```python
from build123d import *

# Parameters (mm, degrees)
SKETCH_1_W           = 58.5
SKETCH_1_H           = 40
EXTRUDE_1_DEPTH      = 25
SKETCH_2_OUTSIDE_W   = 75.53
SKETCH_2_OUTSIDE_H   = 57.03
SKETCH_2_OUTSIDE_W_2 = 51.5
SKETCH_2_OUTSIDE_H_2 = 31.5
CUT_EXTRUDE_4_DEPTH  = 21.5
EXTRUDE_2_REACH      = 45.365
SKETCH_3_W           = 3.457860742
SKETCH_3_H           = 3.97738732
FILLET_1_R           = 3
FILLET_2_R           = 3
FILLET_3_R           = 3


with BuildPart() as part:
    # 草图1 → 凸台-拉伸1 (new body)
    with BuildSketch(Plane.XY):
        Rectangle(SKETCH_1_W, SKETCH_1_H)
    extrude(amount=EXTRUDE_1_DEPTH)

    # 草图2 outside → 切除-拉伸4 (cut)
    with BuildSketch(Plane.XY.offset(25)):
        Rectangle(SKETCH_2_OUTSIDE_W, SKETCH_2_OUTSIDE_H)
        Rectangle(SKETCH_2_OUTSIDE_W_2, SKETCH_2_OUTSIDE_H_2, mode=Mode.SUBTRACT)
    extrude(amount=-CUT_EXTRUDE_4_DEPTH, mode=Mode.SUBTRACT)

    # 草图3 → 凸台-拉伸2 (add, up to next)
    with BuildSketch(Plane.XY.offset(25), mode=Mode.PRIVATE) as extrude_2_sk1:
        with Locations((25.75, 0)):
            Rectangle(SKETCH_3_W, SKETCH_3_H)
    extrude_2_tool1 = extrude(extrude_2_sk1.sketch, amount=-EXTRUDE_2_REACH, mode=Mode.PRIVATE) - part.part
    add(extrude_2_tool1.solids().sort_by_distance((25.75, 0, 25))[0])

    # 圆角1
    fillet_1_edges = [part.edges().sort_by_distance(p)[0] for p in [
        (25.75, -15.75, 14.25),
        (25.75, 15.75, 14.25),
    ]]
    fillet(fillet_1_edges, radius=FILLET_1_R)

    # 圆角2
    fillet_2_edges = [part.edges().sort_by_distance(p)[0] for p in [
        (-25.75, -15.75, 14.25),
        (-25.75, 15.75, 14.25),
    ]]
    fillet(fillet_2_edges, radius=FILLET_2_R)

    # 圆角3
    fillet_3_edges = [part.edges().sort_by_distance(p)[0] for p in [
        (29.25, -20, 1.75),
        (-29.25, -20, 1.75),
        (-29.25, 20, 1.75),
        (29.25, 20, 1.75),
    ]]
    fillet(fillet_3_edges, radius=FILLET_3_R)


solid = part.part
```
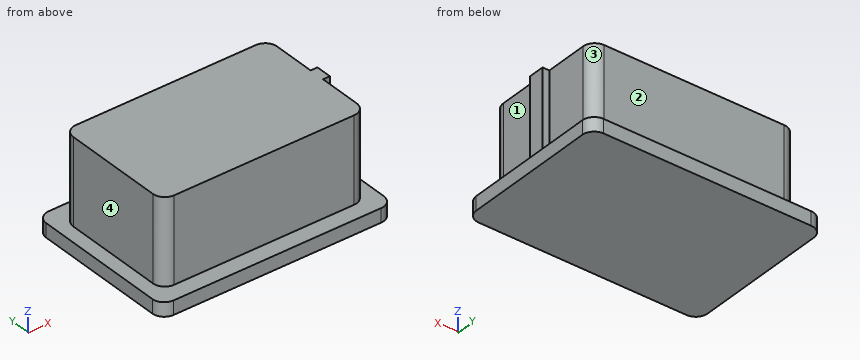
Geometry check sheet. Reference: the model listing, model coordinates, mm. Face numbers are marked on the shaded views. A direction names the side the tool comes from. Coordinates: 2 decimals unless noted, no trailing zeros. Order: outer loops, then holes, each group sorted by start corner. A loop starts at its lowest first (then second) coordinate and runs counter-clockwise, first axis right, second up. Notation, with made-up numbers: (7, 65.5) - (30, 65.5) arc R8 cw to (30, 72.5) - close; hole circle Ø4 at (83, 89). An arc over 180 degrees is marked (long way). Answer in a Markdown table with one row per item. Add a question column.
1. Section check C-C (z = 4.25). Enter the section's corners in (x, y).
2. Material ranges on L1, parallel to Z at x = -26, y = -13; L2, parallel to X at y = 7.5, z = 8; L3, parallel to Y at x = 8, z = 23.5, recorded low to high. Write a range as [from, to].
3. Gauge pin test, flat ends, axial feed: pin 1 Ø1.4 at (x, z) = (26, 10) entering from +Y; pin 2 Ø5.5 at (y, z) = (-8, 9) entering from +X; pin 3 Ø8 at (x, z) = (-9.5, 16) entering from -Y. Record the tip position at first contact, or that the pin passes through.
4. Access from +Z, -Z, +X, -X, +Y, -Y to the whole of each face (thin tool, end or side, straight path). Record for the marked faces 1, 2, 3 and 4.
5. Section check B-B (x = 10). Enter the section's corners in (y, z), plus the area to 3 significant figures.
6. Section check D-D (y = 18). Enter the section's corners in (x, z), plus the area to 3 significant figures.
7. Section check A-A (y = -9). Enter the section's corners in (x, z).
Data:
| question | item | result |
|---|---|---|
| 1 | outline | (-25.75, -12.75) arc R3 ccw to (-22.75, -15.75) - (22.75, -15.75) arc R3 ccw to (25.75, -12.75) - (25.75, -1.99) - (27.48, -1.99) - (27.48, 1.99) - (25.75, 1.99) - (25.75, 12.75) arc R3 ccw to (22.75, 15.75) - (-22.75, 15.75) arc R3 ccw to (-25.75, 12.75) - close |
| 2 | L1 | z = [0, 3.5] |
| 2 | L2 | x = [-25.75, 25.75] |
| 2 | L3 | y = [-15.75, 15.75] |
| 3 | pin 1 | stops at y = 14.33 |
| 3 | pin 2 | stops at x = 25.75 |
| 3 | pin 3 | stops at y = -15.75 |
| 4 | face 1 | +Z, +X, -Y |
| 4 | face 2 | +Z, +X, -X, +Y |
| 4 | face 3 | +Z, +X, +Y |
| 4 | face 4 | +Z, -X, +Y, -Y |
| 5 | outline | (-20, 0) - (20, 0) - (20, 3.5) - (15.75, 3.5) - (15.75, 25) - (-15.75, 25) - (-15.75, 3.5) - (-20, 3.5) - close |
| 5 | area | 817 mm² |
| 6 | outline | (-29.08, 0) - (29.08, 0) - (29.08, 3.5) - (-29.08, 3.5) - close |
| 6 | area | 204 mm² |
| 7 | outline | (-29.25, 0) - (29.25, 0) - (29.25, 3.5) - (25.75, 3.5) - (25.75, 25) - (-25.75, 25) - (-25.75, 3.5) - (-29.25, 3.5) - close |
